Check sheet for the modelled part. Datum: model origin and axes. Units: mm. A direction names the side the tool comes from. Round coordinates to 2 decimals unless told otherwise and drop trailing zeros. Write each loop counter-clockwise with the first axis right and the second up, starting at its lowest first coordinate (ties: lowest second). Pieces come first, ordered by that corner, then holes.
from build123d import *

# Parameters (mm, degrees)
F1_DEPTH      = 350
F1_DEPTH_BACK = 350
F3_D          = 3
F3_DEPTH      = 50
F3_TIP        = 0.9012909285
F4_D          = 3
F4_DEPTH      = 50
F4_START      = 36
F4_TIP        = 0.9012909285


with BuildPart() as f1:
    # F0 (on Right) → F1 (new body, two sides)
    with BuildSketch(Plane.YZ) as f1_sk:
        Polygon((-20, 20), (-20, 0), (20, 0), (20, 20), (18, 20), (18, 2), (-18, 2), (-18, 20), align=None)
    extrude(amount=F1_DEPTH)
    extrude(f1_sk.sketch, amount=-F1_DEPTH_BACK)

    # F3 (one way)
    with BuildSketch(Plane(origin=(0, -18, 0), x_dir=(-1, 0, 0), z_dir=(0, 1, 0))):
        with Locations((-343, 9), (343, 9), (335, 16), (-335, 16)):
            Circle(F3_D / 2)
    extrude(amount=-F3_DEPTH, mode=Mode.SUBTRACT)
    with Locations(Plane(origin=(0, -18, 0), x_dir=(-1, 0, 0), z_dir=(0, 1, 0))):
        with Locations((-343, 9), (343, 9), (335, 16), (-335, 16)):
            with Locations((0, 0, -(F3_DEPTH + F3_TIP / 2))):  # 118° drill point
                Cone(0, F3_D / 2, F3_TIP, mode=Mode.SUBTRACT)

    # F4
    # its depths count from where the whole tool has entered the part; down to there all is cleared
    with Locations(Plane(origin=(0, -18, 0), x_dir=(-1, 0, 0), z_dir=(0, -1, 0)).offset(-F4_START)):
        with Locations((-343, -9), (343, -9), (-335, -16), (335, -16)):
            Hole(F4_D / 2, depth=F4_DEPTH)
            with Locations((0, 0, -(F4_DEPTH + F4_TIP / 2))):  # 118° drill point
                Cone(0, F4_D / 2, F4_TIP, mode=Mode.SUBTRACT)


solid = f1.part
1. Release check for a two-part mould opening along Y. For faces 1 (the flat face through (5, 0, 2)), 2 (the flat face through (5, -20, 10)), 3 (the flat face through (5, 0, 0)) record: released by +Y, released by -Y, zero draft, split by the parting line, or undercut.
2. Set-up check for faces 4 (the flat face through (5, -18, 11)), 5 (the flat face through (-350, 0, 1)): record each of +Z, -Z, +X, -X, +Y, -Y from which the full face is reachable in a straight line by a thin tool's end or side.
3. Sectioned sample at B-B, the plane y = 5. Enter the section's corners in (x, z).
4. Scan lines: line 1 along X through (y, z) = (19.15, 16); line 2 along X through (y, z) = (19.1, 9); line 3 along Z through (x, y) = (-335, 19.05). Record each from-to range of solid material in increasing order.
5. Sectioned sample at A-A, the plane x = -209. Enter the section's corners in (y, z).
6. Go/stop test with flat-tipped pins: pin 1 (4 mm diameter, centred on x = 167.5, y = 12, fed in from -Z); pin 2 (1.8 mm diameter, centred on x = -335, z = 16, fed in from +Y). Record where each tip stops, or that it passes through.
Computed values:
1. face 1: undercut
1. face 2: released by -Y
1. face 3: zero draft
2. face 4: +Z, +X, -X
2. face 5: +Z, -Z, -X, +Y, -Y
3. outline: (-350, 0) - (350, 0) - (350, 2) - (-350, 2) - close
4. line 1: x = -350 to -336.5, -333.5 to 333.5, 336.5 to 350
4. line 2: x = -350 to -344.5, -341.5 to 341.5, 344.5 to 350
4. line 3: z = 0 to 14.5, 17.5 to 20
5. outline: (-20, 0) - (20, 0) - (20, 20) - (18, 20) - (18, 2) - (-18, 2) - (-18, 20) - (-20, 20) - close
6. pin 1: stops at z = 0
6. pin 2: passes through
